from build123d import *

# Parameters (mm, degrees)
SKETCH1_R           = 17.5
BOSS_EXTRUDE1_DEPTH = 5
SKETCH3_R           = 10
BOSS_EXTRUDE2_DEPTH = 50
SKETCH6_R           = 12.5
BOSS_EXTRUDE3_DEPTH = 1
FILLET1_R           = 7.5


with BuildPart() as part:
    # Sketch1 → Boss-Extrude1 (new body)
    with BuildSketch(Plane.XY):
        Circle(SKETCH1_R)
    extrude(amount=BOSS_EXTRUDE1_DEPTH)

    # Sketch3 → Boss-Extrude2 (add)
    with BuildSketch(Plane.XY):
        Circle(SKETCH3_R)
    extrude(amount=BOSS_EXTRUDE2_DEPTH)

    # Sketch6 → Boss-Extrude3 (add)
    with BuildSketch(Plane.XY.offset(50)):
        Circle(SKETCH6_R)
    extrude(amount=BOSS_EXTRUDE3_DEPTH)

    # Sketch7 → Revolve5 (revolve)
    with BuildSketch(Plane.XY.offset(51)):
        with BuildLine():
            Line((0, 12.5), (0, -12.5))
            ThreePointArc((0, -12.5), (-12.5, 0), (0, 12.5))
        make_face()
    revolve(axis=Axis((0, 12.5, 51), (0, -1, 0)))

    # Fillet1
    fillet1_edges = [part.edges().sort_by_distance(p)[0] for p in [
        (-10, 0, 5),
    ]]
    fillet(fillet1_edges, radius=FILLET1_R - 0.0001)  # a hair under: the kernel refuses the full size


solid = part.part
Geometry check sheet. Reference: the model listing, model coordinates, mm. Give positions to 0.01 mm unless a question says otherwise; leave off trailing zeros. Write each loop counter-clockwise with the first axis right and the second up, starting at its lowest first coordinate (ties: lowest second). Pieces come first, ordered by that corner, then holes. Notation, with made-up numbers: M -18,55 L 25,55 A28 cw 25,89 Z; hole C 79.5,11 d11. An arc over 180 degrees is marked long. Answer as CSV lines item,"result". Start each with the question number.
Q1. Material ranges on L1, parallel to Z at x = -7.5, y = -9; L2, parallel to Y at x = 8, z = 41; L3, parallel to Y at x = 6.5, z = 40.5, recorded low to high.
Q2. Section check D-D, the plane z = 52.5. Record the cut outline in (x, y).
Q3. Go/stop test with flat-tipped pins: pin 1 (4 mm diameter, centred on x = -9, z = 56.5, fed in from +Y); pin 2 (10 mm diameter, centred on x = 4, z = 19.5, fed in from +Y); pin 3 (4 mm diameter, centred on y = 11, z = 38.5, fed in from -X). Record where each tip stops, or that it passes through.
Q4. Section check C-C, the plane z = 19. Record the cut outline in (x, y), then the cut area to 3 significant figures.
Q5. Release check for a two-part mould opening along Z. For faces 1 (the face through (-2.17, -9.76, 27.78)), 2 (the face through (-13.887, -10.648, 2.465)), 3 (the face through (0, 0, 0)) record: pulls with the +Z half, pulls with the -Z half, needs draft (parallel to the pull), parting line crosses it, or undercut.
Geometry says:
1,L1,"0 to 7.73, 46.64 to 55.36"
1,L2,"-6 to 6"
1,L3,"-7.6 to 7.6"
2,outline,"C 0,0 d24.82"
3,pin 1,"y = 9.12"
3,pin 2,"y = 10"
3,pin 3,"x = -4.36"
4,outline,"C 0,0 d20"
4,area,"314 mm^2"
5,face 1,"undercut"
5,face 2,"needs draft"
5,face 3,"pulls with the -Z half"
